Design review of the part built by this model. Coordinates are the model's own, in mm. Give positions to 0.01 mm unless a question says otherwise; leave off trailing zeros. Write each loop counter-clockwise with the first axis right and the second up, starting at its lowest first coordinate (ties: lowest second). Pieces come first, ordered by that corner, then holes. Notation, with made-up numbers: M 61.25,-12.5 L 73.25,-12.5 A26 ccw 73.25,14.5 Z; hole C -3.5,50 d4. An arc over 180 degrees is marked long. Use a Markdown table: item, result. Add a question column.
Autodesk Inventor part; units mm, degrees
ref_plane "YZ Plane" through (0, 0, 0) normal (1, 0, 0) x (0, 1, 0)
ref_plane "XZ Plane" through (0, 0, 0) normal (0, 1, 0) x (-1, 0, 0)
ref_plane "XY Plane" through (0, 0, 0) normal (0, 0, 1) x (1, 0, 0)
sketch "スケッチ1" plane through (0, 0, 0) normal (0, 0, 1) x (1, 0, 0)
  line L0 (0, 0) -> (-7.5, 0) construction
  line L1 (0, 3) -> (-7.5, 3)
  line L2 (-7.5, -3) -> (0, -3)
  arc A0 (0, -3) -> (0, 3) centre (0, 0) ccw
  arc A1 (-7.5, 3) -> (-7.5, -3) centre (-7.5, 0) ccw
  circle A2 centre (-7.5, 0) radius 1.5
  circle A3 centre (0, 0) radius 1.5
  line L3 (0, 0) -> (-25, 0) construction
  line L4 (0, -3) -> (-25, -3)
  line L5 (-25, 3) -> (0, 3)
  arc A4 (0, -3) -> (0, 3) centre (0, 0) ccw
  arc A5 (-25, 3) -> (-25, -3) centre (-25, 0) ccw
  circle A6 centre (-25, 0) radius 1.5
  point P0 (-3.75, 0)
  point P1 (-12.5, 0)
  dimension "d0" = 6
  dimension "d1" = 7.5
  dimension "d2" = 3
  dimension "d3" = 3
  dimension "d4" = 25
  dimension "d7" = 3
extrude "押し出し1" add sketch "スケッチ1" along normal blind 3 contours A0 L2 A1 L1 | A1 L4 A5 L5 | A6
properties part number "カウンター先端" material "ポリカーボネート、スモーク"
(1) Add section A-A on x = -7.5. Give the boundary of the cut face in (y, z), then the cut area to 3 significant figures.
(2) Wall thickness on L1, parallel to X at y = 1.2, z = 1.5; L2, parallel to Y at x = -7.5, z = 1.05; L3, parallel to X at y = -0.4, z = 1.3: over which ranges is each line inside the solid? List them lowest first.
(3) The part is to be moulded in two halves that separate along Y. For faces 1 (the flat face through (-13, -3, 1)), 2 (the cylindrical face through (-1.5, -0.07, 1.48)), 3 (the cylindrical face through (3, 0, 1)), say which applies: released by +Y, released by -Y, zero draft, split by the parting line, or undercut.
(4) For pin 1 (2.5 mm diameter, centred on x = -7.5, y = 0, fed in from -Z), flat-tipped, find the tip position at first contact; note if it passes through.
(5) Add section C-C on z = 2.05. Give the boundary of the cut face in (x, y), then the cut area to 3 significant figures.
(6) Add section B-B on y = 0.95. Give the boundary of the cut face in (x, z), then the cut area to 3 significant figures.
(7) Add section D-D on x = -1. Give the boundary of the cut face in (y, z).
From the geometry:
| question | item | result |
|---|---|---|
| 1 | outline | M -3,0 L -1.5,0 L -1.5,3 L -3,3 Z; M 1.5,0 L 3,0 L 3,3 L 1.5,3 Z |
| 1 | area | 9.00 mm^2 |
| 2 | L1 | x = -27.75 to -8.4, -6.6 to -0.9, 0.9 to 2.75 |
| 2 | L2 | y = -3 to -1.5, 1.5 to 3 |
| 2 | L3 | x = -27.97 to -8.95, -6.05 to -1.45, 1.45 to 2.97 |
| 3 | face 1 | released by -Y |
| 3 | face 2 | undercut |
| 3 | face 3 | split by the parting line |
| 4 | pin 1 | passes through |
| 5 | outline | M -25,-3 L 0,-3 A3 ccw 0,3 L -25,3 A3 ccw Z; hole C -7.5,0 d3; hole C 0,0 d3 |
| 5 | area | 164 mm^2 |
| 6 | outline | M -27.85,0 L -8.66,0 L -8.66,3 L -27.85,3 Z; M -6.34,0 L -1.16,0 L -1.16,3 L -6.34,3 Z; M 1.16,0 L 2.85,0 L 2.85,3 L 1.16,3 Z |
| 6 | area | 78.1 mm^2 |
| 7 | outline | M -3,0 L -1.12,0 L -1.12,3 L -3,3 Z; M 1.12,0 L 3,0 L 3,3 L 1.12,3 Z |
